from build123d import *

# Parameters (mm, degrees)
RESSALTO_EXTRUS_O2_DEPTH = 10
FILETE1_R                = 0.3


with BuildPart() as part:
    # Esboço1 → Ressalto-extrusão2 (new body)
    with BuildSketch(Plane(origin=(0, 0, 0), x_dir=(1, 0, 0), z_dir=(0, 1, 0))):
        with BuildLine():
            Line((11.080017789, 84.274748328), (11.262828374, 85.763621058))
            ThreePointArc((11.262828374, 85.763621058), (-0.000523598, 86.499999998), (-11.263866654, 85.763484701))
            Line((-11.263866654, 85.763484701), (-11.081056051, 84.274611816))
            ThreePointArc((-11.081056051, 84.274611816), (-0.000523599, 84.999999998), (11.080017789, 84.274748328))
        make_face()
    extrude(amount=RESSALTO_EXTRUS_O2_DEPTH)

    # Filete1
    filete1_edges = [part.edges().sort_by_distance(p)[0] for p in [
        (-11.081056051, 5, -84.274611816),
        (-11.263866654, 5, -85.763484701),
        (11.262828374, 5, -85.763621058),
        (11.080017789, 5, -84.274748328),
    ]]
    fillet(filete1_edges, radius=FILETE1_R)


solid = part.part
Could you check a few things on this model? Use its own coordinates, in mm. Coordinates: 2 decimals unless noted, no trailing zeros. Write each loop counter-clockwise with the first axis right and the second up, starting at its lowest first coordinate (ties: lowest second). Pieces come first, ordered by that corner, then holes. Notation, with made-up numbers: (-20, -18.75) - (8, -18.75) arc R24 ccw to (8, 4.25) - close; hole circle Ø3 at (-13, 3). An arc over 180 degrees is marked (long way). Write item = value, one per line.
1) Suppose I cut it at B-B on y = 7.5. Please give me the cut outline in (x, z), plus the area to 3 significant figures.
Result set:
outline = (-11.23, -85.47) arc R0.3 ccw to (-10.97, -85.8) arc R86.5 ccw to (10.97, -85.8) arc R0.3 ccw to (11.23, -85.47) - (11.12, -84.57) arc R0.3 ccw to (10.78, -84.31) arc R85 cw to (-10.78, -84.31) arc R0.3 ccw to (-11.12, -84.57) - close
area = 33.5 mm2
2) Will this pin go through, and if not, where does the flat tip stop? pin 1 Ø3 at (x, y) = (-8.5, 6.5) entering from +Z.
Result set:
pin_1 = -84.41
3) Suppose I cut it at D-D on x = -7.5. Please give me the cut outline in (y, z), plus the area to 3 significant figures.
Result set:
outline = (0, -86.17) - (10, -86.17) - (10, -84.67) - (0, -84.67) - close
area = 15.1 mm2
4) Please list where these lines run through material, in increasing order: line 1 (Z direction, x = -0.75, y = 6); line 2 (Z direction, x = -5.25, y = 1); line 3 (X direction, y = 2.5, z = -85.1). Write a range as [from, to].
Result set:
line_1 = [-86.5, -85]
line_2 = [-86.34, -84.84]
line_3 = [-11.18, 11.18]
5) Suppose I cut it at C-C on x = 9.5. Please give me the cut outline in (y, z).
Result set:
outline = (0, -85.98) - (10, -85.98) - (10, -84.47) - (0, -84.47) - close
